Verification items for the finished model (mm, model axes). Face numbers are marked on the shaded views. A direction names the side the tool comes from. Give positions to 0.01 mm unless a question says otherwise; leave off trailing zeros. Loops run counter-clockwise (first coordinate to the right, second up) from the corner with the lowest first, then second, coordinate; pieces in that order, holes last. Notation, with made-up numbers: M -7.5,80 L 28.5,80 A27 ccw 28.5,102 Z; hole C 81.25,59.5 d7. An arc over 180 degrees is marked long. Put each result on its own line as item: value. Start each with the question number.
from build123d import *

# Parameters (mm, degrees)
SKETCH1_W           = 42
SKETCH1_H           = 42
BOSS_EXTRUDE1_DEPTH = 52
SKETCH2_R           = 18
BOSS_EXTRUDE2_DEPTH = 32
SKETCH3_R           = 4
BOSS_EXTRUDE3_DEPTH = 22
SKETCH4_R           = 2.5
BOSS_EXTRUDE4_DEPTH = 11


with BuildPart() as part:
    # Sketch1 → Boss-Extrude1 (new body)
    with BuildSketch(Plane(origin=(0, 0, 0), x_dir=(1, 0, 0), z_dir=(0, 1, 0))):
        Rectangle(SKETCH1_W, SKETCH1_H)
    extrude(amount=BOSS_EXTRUDE1_DEPTH)

    # Sketch2 → Boss-Extrude2 (add)
    with BuildSketch(Plane(origin=(0, 52, 0), x_dir=(1, 0, 0), z_dir=(0, 1, 0))):
        with Locations(Location((0, 0, 0), (0, 0, 270))):
            Circle(SKETCH2_R)
    extrude(amount=BOSS_EXTRUDE2_DEPTH)

    # Sketch3 → Boss-Extrude3 (add)
    with BuildSketch(Plane(origin=(0, 84, 0), x_dir=(1, 0, 0), z_dir=(0, 1, 0))):
        with Locations(Location((0, 0, 0), (0, 0, 270))):
            Circle(SKETCH3_R)
    extrude(amount=BOSS_EXTRUDE3_DEPTH)

    # Sketch4 → Boss-Extrude4 (add)
    with BuildSketch(Plane.XZ):
        with Locations(Location((0, 0, 0), (0, 0, 270))):
            Circle(SKETCH4_R)
    extrude(amount=BOSS_EXTRUDE4_DEPTH)


solid = part.part
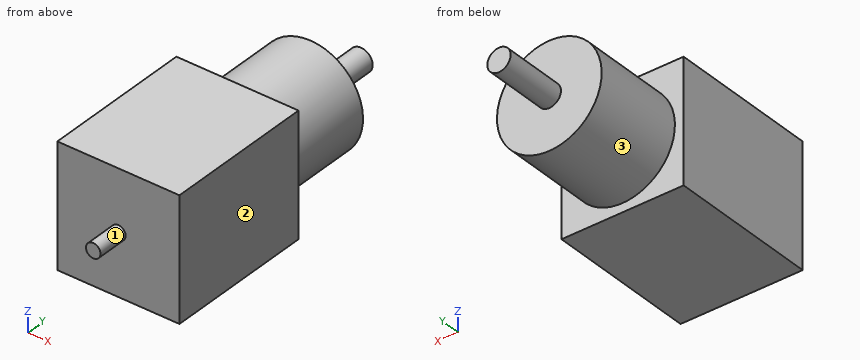
Q1. Cross-section at B-B, the plane x = 0. Record the boundary of the cut face in (y, z).
Q2. Cross-section at C-C, the plane y = 76.5. Record the boundary of the cut face in (x, z), then the cut area to 3 significant figures.
Q3. Cross-section at A-A, the plane z = 0. Record the boundary of the cut face in (x, y), then the cut area to 3 significant figures.
Q4. Scan lines: L1, parallel to Y at x = 10, z = 17; L2, parallel to Y at x = -8.5, z = 6; L3, parallel to Z at x = 11.5, y = 71. Record each from-to range of solid material in increasing order.
Q5. Cross-section at D-D, the plane x = -6. Record the boundary of the cut face in (y, z).
Q6. Set-up check for the marked faces 1, 2 and 3: record each of +Z, -Z, +X, -X, +Y, -Y from which the full face is reachable in a straight line by a thin tool's end or side.
Q7. Go/stop test with flat-tipped pins: pin 1 (18 mm diameter, centred on x = -8.5, z = -6, fed in from +Y); pin 2 (5 mm diameter, centred on y = 81, z = 9, fed in from +X); pin 3 (6 mm diameter, centred on y = 74.5, z = -16, fed in from -X); pin 4 (1 mm diameter, centred on x = 14, z = 12, fed in from -Y). Record where each tip stops, or that it passes through.
Ans:
1. outline: M -11,-2.5 L 0,-2.5 L 0,-21 L 52,-21 L 52,-18 L 84,-18 L 84,-4 L 106,-4 L 106,4 L 84,4 L 84,18 L 52,18 L 52,21 L 0,21 L 0,2.5 L -11,2.5 Z
2. outline: C 0,0 d36
2. area: 1,020 mm^2
3. outline: M -21,0 L -2.5,0 L -2.5,-11 L 2.5,-11 L 2.5,0 L 21,0 L 21,52 L 18,52 L 18,84 L 4,84 L 4,106 L -4,106 L -4,84 L -18,84 L -18,52 L -21,52 Z
3. area: 3,570 mm^2
4. L1: y = 0 to 52
4. L2: y = 0 to 84
4. L3: z = -13.85 to 13.85
5. outline: M 0,-21 L 52,-21 L 52,-16.97 L 84,-16.97 L 84,16.97 L 52,16.97 L 52,21 L 0,21 Z
6. face 1: -Y
6. face 2: +Z, -Z, +X, +Y, -Y
6. face 3: +Y
7. pin 1: stops at y = 106
7. pin 2: stops at x = 16.79
7. pin 3: stops at x = -12.45
7. pin 4: stops at y = 0
